The figure shows three views and two pictorial views of one solid part (mm, origin at its lowest corner). Answer the questions. A direction names the side the tool comes from. Coordinates: 2 decimals unless noted, no trailing zeros. Loops run counter-clockwise (first coordinate to the right, second up) from the corner with the lowest first, then second, coordinate; pieces in that order, holes last. Notation, with made-up numbers: (-12.75, -25.5) -> (-0.75, -25.5) arc R37 cw to (-0.75, 11.5) -> close; hole circle Ø1 at (29.5, -7.75). An arc over 180 degrees is marked (long way). Answer as a JSON object with one key per item and string values. Group by question number.
1) Section C-C, the plane x = 2.25 is taken. Give the vertices of the cut face in (y, z) (1 decimal).
2) Consider probe 1 along Z at (x, y) = (12.5, 0.45); probe 2 along Y at (x, z) = (0.5, 5); probe 3 along X at (y, z) = (1.4, 5). Determine where each line is inside the solid, lowest interval first. Write a range as [from, to].
3) Which of the six approach directions +Z, -Z, +X, -X, +Y, -Y give full straight-line access (tool end or side, diameter ignored) to the marked faces 1 and 2?
4) Determine the mould class of the marked faces 3, 4, 5 and 6 for opening direction Z: released by +Z, released by -Z, zero draft, split by the parting line, or undercut.
5) Section D-D, the plane z = 1 is taken. Give the vertices of the cut face in (x, y), plus the area to 3 significant figures.
6) Section A-A, the plane x = 12.5 is taken. Give the vertices of the cut face in (y, z).
7) Flat-ended cylindrical pins translate along their axes: P1, Ø4, axis at x = 12.5, z = 5, coming from the +Y side; P2, Ø4.5, axis at y = 11, z = 3.5, coming from the +X side; P3, Ø4, axis at y = 12.5, z = 5, coming from the +X side. Find the tip coordinate at first contact, or state that the pin passes through.
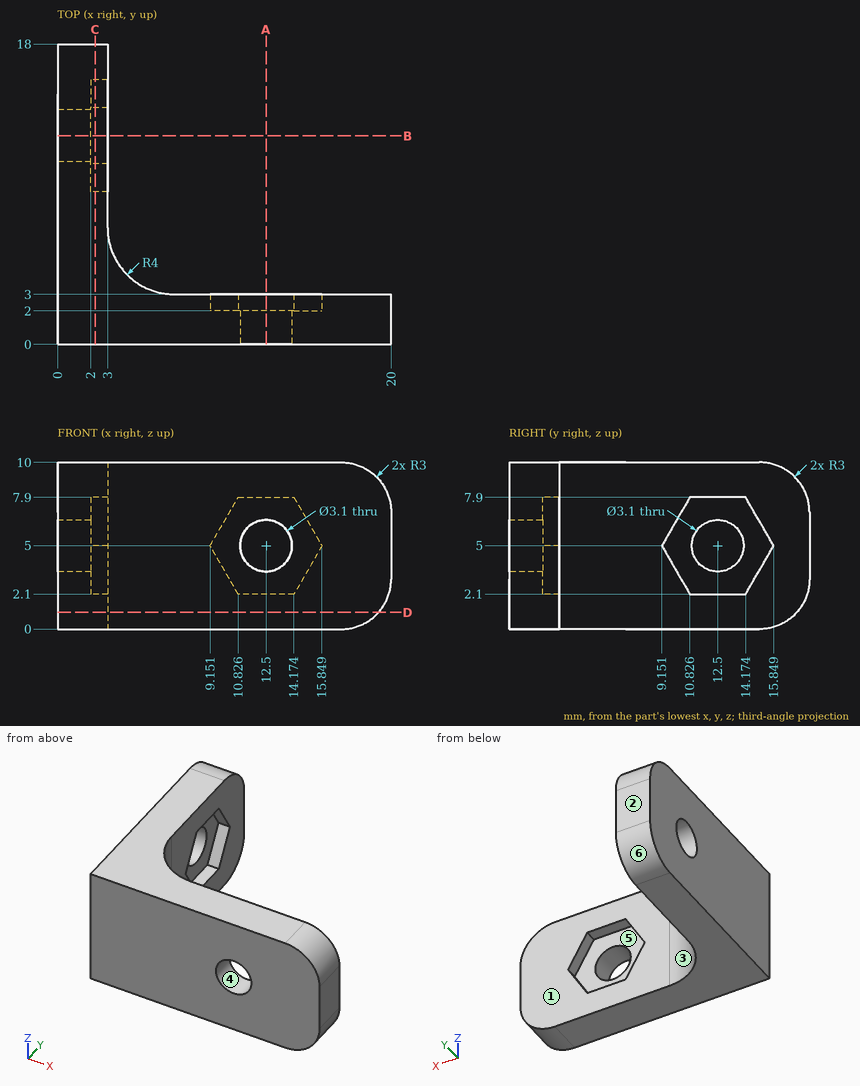
Determined:
{
 "1": {"outline": "(0, 0) -> (15, 0) arc R3 ccw to (18, 3) -> (18, 7) arc R3 ccw to (15, 10) -> (0, 10) -> close; hole (9.2, 5) -> (10.8, 2.1) -> (14.2, 2.1) -> (15.8, 5) -> (14.2, 7.9) -> (10.8, 7.9) -> close"},
 "2": {"probe 1": "[0, 3.45], [6.55, 10]", "probe 2": "[0, 10.95], [14.05, 18]", "probe 3": "[0, 10.95], [14.05, 20]"},
 "3": {"face 1": "+Z, -Z, +X, +Y", "face 2": "+Z, -Z, +X, -X, +Y"},
 "4": {"face 3": "zero draft", "face 4": "undercut", "face 5": "undercut", "face 6": "released by -Z"},
 "5": {"outline": "(0, 0) -> (19.24, 0) -> (19.24, 3) -> (7, 3) arc R4 cw to (3, 7) -> (3, 17.24) -> (0, 17.24) -> close", "area": "104 mm²"},
 "6": {"outline": "(0, 0) -> (3, 0) -> (3, 2.1) -> (2, 2.1) -> (2, 3.45) -> (0, 3.45) -> close; (0, 6.55) -> (2, 6.55) -> (2, 7.9) -> (3, 7.9) -> (3, 10) -> (0, 10) -> close"},
 "7": {"P1": "y = 2", "P2": "x = 3", "P3": "x = 2"}
}
